from build123d import *

# Parameters (mm, degrees)
CHAMFER2_SIZE      = 0.5
CUT_EXTRUDE1_DEPTH = 2


with BuildPart() as part:
    # Sketch1 → Revolve1 (revolve)
    with BuildSketch(Plane.XY):
        Polygon((0, 3), (60, 3), (60, 1.5), (62, 1.5), (62, 2), (67, 2), (67, 0), (-4, 0), (-4, 4.5), (0, 4.5), align=None)
    revolve(axis=Axis((-15.448246648, 0, 0), (1, 0, 0)))

    # Chamfer2
    chamfer2_edges = [part.edges().sort_by_distance(p)[0] for p in [
        (-4, -4.5, 0),
    ]]
    chamfer(chamfer2_edges, length=CHAMFER2_SIZE)

    # Sketch2 → Cut-Extrude1 (cut)
    with BuildSketch(Plane.ZY.offset(4)):
        Polygon((0, 1.732050808), (-1.5, 0.866025404), (-1.5, -0.866025404), (0, -1.732050808), (1.5, -0.866025404), (1.5, 0.866025404), align=None)
    extrude(amount=-CUT_EXTRUDE1_DEPTH, mode=Mode.SUBTRACT)


solid = part.part
Work out the finished part from the listing and answer in its coordinate system (mm). A direction names the side the tool comes from. Round coordinates to 2 decimals unless told otherwise and drop trailing zeros. Loops run counter-clockwise (first coordinate to the right, second up) from the corner with the lowest first, then second, coordinate; pieces in that order, holes last. Notation, with made-up numbers: M 14.5,-9.75 L 46.5,-9.75 A13 cw 46.5,9.25 Z; hole C 31.5,-12 d9. An arc over 180 degrees is marked long. One line per question, with ' | ' between items. Start each with the question number.
(1) Flat-ended cylindrical pins translate along their axes: pin 1 Ø1.2 at (y, z) = (0, 0.5) entering from -X; pin 2 Ø4 at (x, z) = (28.5, -1.5) entering from -Y; pin 3 Ø5 at (x, y) = (47.5, 2.5) entering from -Z. Find the tip coordinate at first contact, or state that the pin passes through.
(2) A cutting plane is placed at B-B on x = 30. Write down the section's boundary in (y, z), plus the area to 3 significant figures.
(3) Find the intervals of material crossed by line 1 (X direction, y = 1.25, z = 1.5); line 2 (X direction, y = 2, z = -2.75); line 3 (X direction, y = 0.75, z = 0), in increasing order.
(4) For a pull along Y with two mould halves and no side action, classify faces 5 (the face through (60, 1.3, -1.3)), 6 (the face through (-3.014, -1.293, -0.76)), 7 (the face through (65, 0, -2)) as released by +Y, released by -Y, zero draft, split by the parting line, or undercut.
(5) A cutting plane is placed at A-A on y = 0. Write down the section's boundary in (x, z).
(6) A tool of negligible diameter and unlimited length cuts with its end or side. For faces 1 (the face through (-1.73, -0.59, 4.46)), 2 (the face through (30, -3, 0)), 3 (the face through (61.01, -1.5, 0.07)), 4 (the face through (-3, 0, 1.5)), from which of +Z, -Z, +X, -X, +Y, -Y can it reach the whole face along a straight path? Write none if from no direction.
Geometry check:
1) pin 1: stops at x = -2 | pin 2: stops at y = -3 | pin 3: stops at z = -3
2) outline: C 0,0 d6 | area: 28.3 mm²
3) line 1: x = -4 to 60, 62 to 67 | line 2: x = -4 to 0 | line 3: x = -2 to 67
4) face 5: zero draft | face 6: undercut | face 7: split by the parting line
5) outline: M -4,-4 L -3.5,-4.5 L 0,-4.5 L 0,-3 L 60,-3 L 60,-1.5 L 62,-1.5 L 62,-2 L 67,-2 L 67,2 L 62,2 L 62,1.5 L 60,1.5 L 60,3 L 0,3 L 0,4.5 L -3.5,4.5 L -4,4 L -4,1.5 L -2,1.5 L -2,-1.5 L -4,-1.5 Z
6) face 1: +X, -X | face 2: +X | face 3: none | face 4: -X
